Here's how the part is built. I have some questions about the finished solid (model axes, mm). A direction names the side the tool comes from. Coordinates: 2 decimals unless noted, no trailing zeros. Loops run counter-clockwise (first coordinate to the right, second up) from the corner with the lowest first, then second, coordinate; pieces in that order, holes last. Notation, with made-up numbers: (55, 72.5) -> (113, 72.5) arc R31 cw to (113, 106.5) -> close; hole circle Ø7 at (0, -26). An arc over 180 degrees is marked (long way). Answer as a JSON object with one key per item and string values. Group by question number.
Q1. I'm going to push flat-ended pins straight in: pin 1 (7 mm diameter, centred on x = 46.5, z = 1.5, fed in from -Y); pin 2 (12 mm diameter, centred on x = 49.5, y = 34, fed in from -Z); pin 3 (8 mm diameter, centred on y = 41.5, z = -4.5, fed in from +X); pin 4 (6 mm diameter, centred on y = 31.5, z = 2.5, fed in from +X). Where does each tip first touch, or does it pass through?
Q2. On a 3-axis mill with a long thin cutter (end or side, diameter ignored), from which of +Z, -Z, +X, -X, +Y, -Y can I reach the whole of each face in a straight line? I mean faces 1 (the flat face through (38, 21.35, 0)), 2 (the flat face through (80, 5, -6.5)). Say none if no direction works.
Q3. I want a section at B-B on x = 92. Write out the boundary of the cut face in (y, z).
Q4. Thinking about a two-plate mould opening in X: for faces 3 (the cylindrical face through (64.36, 24.39, 0.46)), 4 (the flat face through (72, 44, -5)), 5 (the flat face through (38, 13, -2.2)), which applies, released by +X, released by -X, zero draft, split by the parting line, or undercut?
Q5. I want a section at D-D on x = 82.5. Write out the boundary of the cut face in (y, z).
Q6. I want a section at C-C on z = -5.75. Write out the boundary of the cut face in (x, y).
Q7. I want a section at A-A on y = 13. Write out the boundary of the cut face in (x, z), then the cut area to 3 significant figures.
Q8. I need wall thicknesses on line 1 (Y direction, x = 92, z = -4.25); line 2 (X direction, y = 44.8, z = 0); line 3 (X direction, y = 25.6, z = 0). Which ranges of each line are inside material? Lowest first, please.
```python
from build123d import *

# Parameters (mm, degrees)
BOSS_EXTRUDE1_START  = 17.075
SKETCH1_W            = 32.8
SKETCH1_H            = 16.2
BOSS_EXTRUDE1_DEPTH  = 10.275
BOSS_EXTRUDE2_START  = 5
SKETCH2_W            = 31
SKETCH2_H            = 12.1
BOSS_EXTRUDE2_DEPTH  = 1.5
BOSS_EXTRUDE3_START  = 5
SKETCH3_W            = 16
SKETCH3_H            = 14.6
BOSS_EXTRUDE3_DEPTH  = 1.5
BOSS_EXTRUDE4_START  = 5
SKETCH4_W            = 10.5
SKETCH4_H            = 8.1
BOSS_EXTRUDE4_DEPTH  = 1.5
BOSS_EXTRUDE5_START  = 5
SKETCH5_R            = 6.5
BOSS_EXTRUDE5_DEPTH  = 1.5
CUT_EXTRUDE1_START   = 5
SKETCH6_R            = 2.95
CUT_EXTRUDE1_DEPTH   = 1.5
BOSS_EXTRUDE6_START  = 70.2
SKETCH7_W            = 12.1
SKETCH7_H            = 42.2
BOSS_EXTRUDE6_DEPTH  = 2
BOSS_EXTRUDE7_START  = 68.05
SKETCH8_W            = 12.1
SKETCH8_H            = 20.55
BOSS_EXTRUDE7_DEPTH  = 1.15
BOSS_EXTRUDE8_START  = 43.6
SKETCH9_W            = 19.8
SKETCH9_H            = 12.1
BOSS_EXTRUDE8_DEPTH  = 2.1
BOSS_EXTRUDE9_START  = 43.6
SKETCH10_W           = 16
SKETCH10_H           = 14.6
BOSS_EXTRUDE9_DEPTH  = 2.1
BOSS_EXTRUDE10_START = 43.6
SKETCH11_W           = 10.5
SKETCH11_H           = 8.1
BOSS_EXTRUDE10_DEPTH = 2.1
BOSS_EXTRUDE11_START = 43.6
SKETCH12_R           = 6.5
BOSS_EXTRUDE11_DEPTH = 2.1
CUT_EXTRUDE2_START   = 43.6
SKETCH13_R           = 3.55
CUT_EXTRUDE2_DEPTH   = 2.1
CUT_EXTRUDE3_START   = 43.6
CUT_EXTRUDE3_DEPTH   = 2.1
CUT_EXTRUDE4_START   = 18.725
SKETCH15_W           = 23.2
SKETCH15_H           = 13
CUT_EXTRUDE4_DEPTH   = 8.625
CUT_EXTRUDE5_START   = 24.35
SKETCH16_R           = 1
CUT_EXTRUDE5_DEPTH   = 3
CUT_EXTRUDE6_START   = 24.35
SKETCH17_R           = 1
CUT_EXTRUDE6_DEPTH   = 3
CUT_EXTRUDE7_START   = 8.1
SKETCH18_R           = 3.15
CUT_EXTRUDE7_DEPTH   = 1.3
CUT_EXTRUDE8_START   = 37.5
SKETCH19_W           = 4.4
SKETCH19_H           = 6
CUT_EXTRUDE8_DEPTH   = 2.4


with BuildPart() as part:
    # Sketch1 → Boss-Extrude1 (new, symmetric)
    with BuildSketch(Plane(origin=(0, 0, 0), x_dir=(1, 0, 0), z_dir=(0, 1, 0)).offset(BOSS_EXTRUDE1_START)):
        with Locations((51.5, 0)):
            Rectangle(SKETCH1_W, SKETCH1_H)
    extrude(amount=BOSS_EXTRUDE1_DEPTH, both=True)



with BuildPart() as body_2:
    # Sketch2 → Boss-Extrude2 (new, symmetric)
    with BuildSketch(Plane(origin=(0, 0, 0), x_dir=(1, 0, 0), z_dir=(0, 1, 0)).offset(BOSS_EXTRUDE2_START)):
        with Locations((72.5, -2.05)):
            Rectangle(SKETCH2_W, SKETCH2_H)
    extrude(amount=BOSS_EXTRUDE2_DEPTH, both=True)

    # Sketch3 → Boss-Extrude3 (add, symmetric)
    with BuildSketch(Plane(origin=(0, 0, 0), x_dir=(1, 0, 0), z_dir=(0, 1, 0)).offset(BOSS_EXTRUDE3_START)):
        with Locations((80, -0.8)):
            Rectangle(SKETCH3_W, SKETCH3_H)
    extrude(amount=BOSS_EXTRUDE3_DEPTH, both=True)

    # Sketch4 → Boss-Extrude4 (add, symmetric)
    with BuildSketch(Plane(origin=(0, 0, 0), x_dir=(1, 0, 0), z_dir=(0, 1, 0)).offset(BOSS_EXTRUDE4_START)):
        with Locations((93.25, -4.05)):
            Rectangle(SKETCH4_W, SKETCH4_H)
    extrude(amount=BOSS_EXTRUDE4_DEPTH, both=True)

    # Sketch5 → Boss-Extrude5 (add, symmetric)
    with BuildSketch(Plane(origin=(0, 0, 0), x_dir=(1, 0, 0), z_dir=(0, 1, 0)).offset(BOSS_EXTRUDE5_START)):
        with Locations((92, 0)):
            Circle(SKETCH5_R)
    extrude(amount=BOSS_EXTRUDE5_DEPTH, both=True)

    # Sketch6 → Cut-Extrude1 (cut, symmetric)
    with BuildSketch(Plane(origin=(0, 0, 0), x_dir=(1, 0, 0), z_dir=(0, 1, 0)).offset(CUT_EXTRUDE1_START)):
        with Locations(Location((92, 0, 0), (0, 0, 270))):
            Circle(SKETCH6_R)
    extrude(amount=CUT_EXTRUDE1_DEPTH, both=True, mode=Mode.SUBTRACT)

    # Sketch7 → Boss-Extrude6 (add, symmetric)
    with BuildSketch(Plane(origin=(0, 0, 0), x_dir=(0, 0, -1), z_dir=(1, 0, 0)).offset(BOSS_EXTRUDE6_START)):
        with Locations((-2.05, 24.6)):
            Rectangle(SKETCH7_W, SKETCH7_H)
    extrude(amount=BOSS_EXTRUDE6_DEPTH, both=True)


with BuildPart() as part_1:
    add(part.part)

    add(body_2.part)  # Boss-Extrude7 merges body 2
    # Sketch8 → Boss-Extrude7 (add, symmetric)
    with BuildSketch(Plane(origin=(0, 0, 0), x_dir=(0, 0, -1), z_dir=(1, 0, 0)).offset(BOSS_EXTRUDE7_START)):
        with Locations((-2.05, 17.075)):
            Rectangle(SKETCH8_W, SKETCH8_H)
    extrude(amount=BOSS_EXTRUDE7_DEPTH, both=True)

    # Sketch9 → Boss-Extrude8 (add, symmetric)
    with BuildSketch(Plane(origin=(0, 0, 0), x_dir=(1, 0, 0), z_dir=(0, 1, 0)).offset(BOSS_EXTRUDE8_START)):
        with Locations((78.1, -2.05)):
            Rectangle(SKETCH9_W, SKETCH9_H)
    extrude(amount=BOSS_EXTRUDE8_DEPTH, both=True)

    # Sketch10 → Boss-Extrude9 (add, symmetric)
    with BuildSketch(Plane(origin=(0, 0, 0), x_dir=(1, 0, 0), z_dir=(0, 1, 0)).offset(BOSS_EXTRUDE9_START)):
        with Locations((80, -0.8)):
            Rectangle(SKETCH10_W, SKETCH10_H)
    extrude(amount=BOSS_EXTRUDE9_DEPTH, both=True)

    # Sketch11 → Boss-Extrude10 (add, symmetric)
    with BuildSketch(Plane(origin=(0, 0, 0), x_dir=(1, 0, 0), z_dir=(0, 1, 0)).offset(BOSS_EXTRUDE10_START)):
        with Locations((93.25, -4.05)):
            Rectangle(SKETCH11_W, SKETCH11_H)
    extrude(amount=BOSS_EXTRUDE10_DEPTH, both=True)

    # Sketch12 → Boss-Extrude11 (add, symmetric)
    with BuildSketch(Plane(origin=(0, 0, 0), x_dir=(1, 0, 0), z_dir=(0, 1, 0)).offset(BOSS_EXTRUDE11_START)):
        with Locations((92, 0)):
            Circle(SKETCH12_R)
    extrude(amount=BOSS_EXTRUDE11_DEPTH, both=True)

    # Sketch13 → Cut-Extrude2 (cut, symmetric)
    with BuildSketch(Plane(origin=(0, 0, 0), x_dir=(1, 0, 0), z_dir=(0, 1, 0)).offset(CUT_EXTRUDE2_START)):
        with Locations(Location((92, 0, 0), (0, 0, 270))):
            Circle(SKETCH13_R)
    extrude(amount=CUT_EXTRUDE2_DEPTH, both=True, mode=Mode.SUBTRACT)

    # Sketch14 → Cut-Extrude3 (cut, symmetric)
    with BuildSketch(Plane(origin=(0, 0, 0), x_dir=(1, 0, 0), z_dir=(0, 1, 0)).offset(CUT_EXTRUDE3_START)):
        Polygon((92, 3.55), (79.3, 2.403281405), (79.3, -2.403281405), (92, -3.55), align=None)
    extrude(amount=CUT_EXTRUDE3_DEPTH, both=True, mode=Mode.SUBTRACT)

    # Sketch15 → Cut-Extrude4 (cut, symmetric)
    with BuildSketch(Plane(origin=(0, 0, 0), x_dir=(1, 0, 0), z_dir=(0, 1, 0)).offset(CUT_EXTRUDE4_START)):
        with Locations((51.5, 0)):
            Rectangle(SKETCH15_W, SKETCH15_H)
    extrude(amount=CUT_EXTRUDE4_DEPTH, both=True, mode=Mode.SUBTRACT)

    # Sketch16 → Cut-Extrude5 (cut, symmetric)
    with BuildSketch(Plane(origin=(0, 0, 0), x_dir=(1, 0, 0), z_dir=(0, 1, 0)).offset(CUT_EXTRUDE5_START)):
        with Locations(Location((65.25, 0, 0), (0, 0, 270))):
            Circle(SKETCH16_R)
    extrude(amount=CUT_EXTRUDE5_DEPTH, both=True, mode=Mode.SUBTRACT)

    # Sketch17 → Cut-Extrude6 (cut, symmetric)
    with BuildSketch(Plane(origin=(0, 0, 0), x_dir=(1, 0, 0), z_dir=(0, 1, 0)).offset(CUT_EXTRUDE6_START)):
        with Locations(Location((37.75, 0, 0), (0, 0, 270))):
            Circle(SKETCH17_R)
    extrude(amount=CUT_EXTRUDE6_DEPTH, both=True, mode=Mode.SUBTRACT)

    # Sketch18 → Cut-Extrude7 (cut, symmetric)
    with BuildSketch(Plane(origin=(0, 0, 0), x_dir=(1, 0, 0), z_dir=(0, 1, 0)).offset(CUT_EXTRUDE7_START)):
        with Locations(Location((46, 0, 0), (0, 0, 270))):
            Circle(SKETCH18_R)
    extrude(amount=CUT_EXTRUDE7_DEPTH, both=True, mode=Mode.SUBTRACT)

    # Sketch19 → Cut-Extrude8 (cut, symmetric)
    with BuildSketch(Plane(origin=(0, 0, 0), x_dir=(0, 0, -1), z_dir=(1, 0, 0)).offset(CUT_EXTRUDE8_START)):
        with Locations((0, 13.1)):
            Rectangle(SKETCH19_W, SKETCH19_H)
    extrude(amount=CUT_EXTRUDE8_DEPTH, both=True, mode=Mode.SUBTRACT)


solid = part_1.part
```
Result set:
{
 "1": {"pin 1": "stops at y = 6.8", "pin 2": "passes through", "pin 3": "stops at x = 98.48", "pin 4": "stops at x = 72.2"},
 "2": {"face 1": "+Y", "face 2": "-Z, +X, -X, +Y, -Y"},
 "3": {"outline": "(3.5, -6.5) -> (6.5, -6.5) -> (6.5, -2.95) -> (3.5, -2.95) -> close; (3.5, 2.95) -> (6.5, 2.95) -> (6.5, 8.1) -> (3.5, 8.1) -> close; (41.5, -6.5) -> (45.7, -6.5) -> (45.7, -3.55) -> (41.5, -3.55) -> close; (41.5, 3.55) -> (45.7, 3.55) -> (45.7, 8.1) -> (41.5, 8.1) -> close"},
 "4": {"face 3": "undercut", "face 4": "released by -X", "face 5": "zero draft"},
 "5": {"outline": "(3.5, -6.5) -> (6.5, -6.5) -> (6.5, 8.1) -> (3.5, 8.1) -> close; (41.5, -6.5) -> (45.7, -6.5) -> (45.7, -2.69) -> (41.5, -2.69) -> close; (41.5, 2.69) -> (45.7, 2.69) -> (45.7, 8.1) -> (41.5, 8.1) -> close"},
 "6": {"outline": "(35.1, 6.8) -> (67.9, 6.8) -> (67.9, 27.35) -> (63.1, 27.35) -> (63.1, 10.1) -> (39.9, 10.1) -> (39.9, 27.35) -> (35.1, 27.35) -> close; (72, 3.5) -> (88, 3.5) -> (88, 6.5) -> (72, 6.5) -> close; (72, 41.5) -> (88, 41.5) -> (88, 45.7) -> (72, 45.7) -> close; (88.97, 3.5) -> (95.03, 3.5) -> (95.03, 6.5) -> (88.97, 6.5) -> close; (88.97, 41.5) -> (95.03, 41.5) -> (95.03, 45.7) -> (88.97, 45.7) -> close"},
 "7": {"outline": "(35.1, -8.1) -> (67.9, -8.1) -> (67.9, -4) -> (72.2, -4) -> (72.2, 8.1) -> (35.1, 8.1) -> (35.1, 2.2) -> (39.9, 2.2) -> (39.9, 6.5) -> (63.1, 6.5) -> (63.1, -6.5) -> (39.9, -6.5) -> (39.9, -2.2) -> (35.1, -2.2) -> close", "area": "261 mm²"},
 "8": {"line 1": "y = 3.5 to 6.5, 41.5 to 45.7", "line 2": "x = 68.2 to 79.3, 95.55 to 98.5", "line 3": "x = 35.1 to 36.75, 38.75 to 39.9, 63.1 to 64.25, 66.25 to 72.2"}
}
